Part model, mm, in its own coordinate system. A direction names the side the tool comes from. Coordinates: 2 decimals unless noted, no trailing zeros. Loops run counter-clockwise (first coordinate to the right, second up) from the corner with the lowest first, then second, coordinate; pieces in that order, holes last. Notation, with made-up numbers: (48.5, -22.5) - (90.5, -22.5) arc R13 cw to (90.5, -6.5) - close; hole circle Ø2 at (-22, 63). An arc over 180 degrees is marked (long way). Use a Markdown table: item, result. Add a question column.
1. Pull direction Z, two halves, no side cores. Call faces 4 (the flat face through (17, 30, 13)), 5 (the flat face through (73, 69, 3)), 6 (the cylindrical face through (57.846, 49.451, 7.93)): pulls with the +Z half, pulls with the -Z half, needs draft (parallel to the pull), parting line crosses it, or undercut.
2. Band-saw the part on D-D, the plane z = 19.5. Give the cut face in (x, y).
3. Band-saw the part on A-A, the plane x = 96. Give the cut face in (y, z).
4. Band-saw the part on C-C, the plane x = 154. Give the cut face in (y, z).
5. Wall check: probe 1 along Y at (x, z) = (8, 1.25); probe 2 along X at (y, z) = (29, 10); probe 3 along X at (y, z) = (56, 1). Give the ranges that are in metal, low to high. Write a range as [from, to].
6. 3-axis set-ups, long thin cutter, end or side, ignore diameter. For faces 1 (the flat face through (25, 98, 25)), 2 (the flat face through (56, 52, 13)), 3 (the cylindrical face through (107.05, 22.7, 7.93)): which of +Z, -Z, +X, -X, +Y, -Y reach the whole face in a straight line?
7. Band-saw the part on B-B, the plane x = 64.5. Give the cut face in (y, z).
8. Drop flat-ended pins along their axis: pin 1 (2 mm diameter, centred on x = 143, z = 41.5, fed in from +Y); pin 2 (1.5 mm diameter, centred on y = 67, z = 1.5, fed in from +X); pin 3 (21.5 mm diameter, centred on y = 92.5, z = 35.5, fed in from -X). Give the stop position or say it passes through.
from build123d import *

# Parameters (mm, degrees)
BOX006_W                  = 35
BOX006_H                  = 25
BOX006_DEPTH              = 10
CYLINDER010_R             = 0.7
CYLINDER010_DEPTH         = 10
CYLINDER011_R             = 4
CYLINDER011_DEPTH         = 10
CYLINDER012_R             = 0.7
CYLINDER012_DEPTH         = 10
CYLINDER013_R             = 4
CYLINDER013_DEPTH         = 10
CYLINDER009_R             = 0.7
CYLINDER009_DEPTH         = 10
CYLINDER008_R             = 4
CYLINDER008_DEPTH         = 10
CYLINDER016_R             = 0.7
CYLINDER016_DEPTH         = 10
CYLINDER017_R             = 4
CYLINDER017_DEPTH         = 10
CYLINDER018_R             = 0.7
CYLINDER018_DEPTH         = 10
CYLINDER019_R             = 4
CYLINDER019_DEPTH         = 10
FUSION003_PLACEMENT_ANGLE = 90
CYLINDER006_R             = 1
CYLINDER006_DEPTH         = 10
CYLINDER007_R             = 1
CYLINDER007_DEPTH         = 10
BOX005_W                  = 142
BOX005_H                  = 54
BOX005_DEPTH              = 3
CUT010_PLACEMENT_ANGLE    = 62
CYLINDER_R                = 1.5
CYLINDER_DEPTH            = 10
CYLINDER001_R             = 1.5
CYLINDER001_DEPTH         = 10
CYLINDER002_R             = 1.5
CYLINDER002_DEPTH         = 10
CYLINDER003_R             = 1.5
CYLINDER003_DEPTH         = 10
CYLINDER004_R             = 1.5
CYLINDER004_DEPTH         = 10
CYLINDER005_R             = 1.5
CYLINDER005_DEPTH         = 10
BOX004_W                  = 76
BOX004_H                  = 76
BOX004_DEPTH              = 10
BOX002_W                  = 192
BOX002_H                  = 72
BOX002_DEPTH              = 3
BOX003_W                  = 172
BOX003_H                  = 112
BOX003_DEPTH              = 3
BOX001_W                  = 192
BOX001_H                  = 112
BOX001_DEPTH              = 3
BOX_W                     = 192
BOX_H                     = 112
BOX_DEPTH                 = 3


with BuildPart() as cube006:
    # Box006 → Box006 (new body)
    with BuildSketch(Plane(origin=(81, 36, 0), x_dir=(1, 0, 0), z_dir=(0, 0, 1))):
        with Locations((17.5, 12.5)):
            Rectangle(BOX006_W, BOX006_H)
    extrude(amount=BOX006_DEPTH)


with BuildPart() as cylinder010:
    # Cylinder010 → Cylinder010 (new body)
    with BuildSketch(Plane.XY.offset(3)):
        Circle(CYLINDER010_R)
    extrude(amount=CYLINDER010_DEPTH)


with BuildPart() as cut012:
    # Cylinder011 → Cylinder011 (new body)
    with BuildSketch(Plane.XY.offset(3)):
        Circle(CYLINDER011_R)
    extrude(amount=CYLINDER011_DEPTH)

    # Cut012: cut Cylinder010
    add(cylinder010.part, mode=Mode.SUBTRACT)


with BuildPart() as cut012_1:
    # Cut012 placement: moved
    add(cut012.part.moved(Location((0, 34, 0))))


with BuildPart() as cylinder012:
    # Cylinder012 → Cylinder012 (new body)
    with BuildSketch(Plane.XY.offset(3)):
        Circle(CYLINDER012_R)
    extrude(amount=CYLINDER012_DEPTH)


with BuildPart() as cut013:
    # Cylinder013 → Cylinder013 (new body)
    with BuildSketch(Plane.XY.offset(3)):
        Circle(CYLINDER013_R)
    extrude(amount=CYLINDER013_DEPTH)

    # Cut013: cut Cylinder012
    add(cylinder012.part, mode=Mode.SUBTRACT)


with BuildPart() as cut013_1:
    # Cut013 placement: moved
    add(cut013.part.moved(Location((54, 1, 0))))


with BuildPart() as cylinder009:
    # Cylinder009 → Cylinder009 (new body)
    with BuildSketch(Plane.XY.offset(3)):
        Circle(CYLINDER009_R)
    extrude(amount=CYLINDER009_DEPTH)


with BuildPart() as fusion002:
    # Cylinder008 → Cylinder008 (new body)
    with BuildSketch(Plane.XY.offset(3)):
        Circle(CYLINDER008_R)
    extrude(amount=CYLINDER008_DEPTH)

    # Cut011: cut Cylinder009
    add(cylinder009.part, mode=Mode.SUBTRACT)

    # Fusion002: union Cut012, Cut013
    add(cut012_1.part)
    add(cut013_1.part)


with BuildPart() as fusion002_1:
    # Fusion002 placement: moved
    add(fusion002.part.moved(Location((56, 19, 0))))


with BuildPart() as cylinder016:
    # Cylinder016 → Cylinder016 (new body)
    with BuildSketch(Plane.XY.offset(3)):
        Circle(CYLINDER016_R)
    extrude(amount=CYLINDER016_DEPTH)


with BuildPart() as cut015:
    # Cylinder017 → Cylinder017 (new body)
    with BuildSketch(Plane.XY.offset(3)):
        Circle(CYLINDER017_R)
    extrude(amount=CYLINDER017_DEPTH)

    # Cut015: cut Cylinder016
    add(cylinder016.part, mode=Mode.SUBTRACT)


with BuildPart() as cut015_1:
    # Cut015 placement: moved
    add(cut015.part.moved(Location((0, 16, 0))))


with BuildPart() as cylinder018:
    # Cylinder018 → Cylinder018 (new body)
    with BuildSketch(Plane.XY.offset(3)):
        Circle(CYLINDER018_R)
    extrude(amount=CYLINDER018_DEPTH)


with BuildPart() as fusion003:
    # Cylinder019 → Cylinder019 (new body)
    with BuildSketch(Plane.XY.offset(3)):
        Circle(CYLINDER019_R)
    extrude(amount=CYLINDER019_DEPTH)

    # Cut016: cut Cylinder018
    add(cylinder018.part, mode=Mode.SUBTRACT)


with BuildPart() as fusion003_1:
    # Cut016 placement: moved
    add(fusion003.part.moved(Location((30, 0, 0))))

    # Fusion003: union Cut015
    add(cut015_1.part)


with BuildPart() as fusion003_2:
    # Fusion003 placement: moved
    add(fusion003_1.part.moved(Location((33, 29, 0))).rotate(Axis((33, 29, 0), (0, 0, 1)), FUSION003_PLACEMENT_ANGLE))


with BuildPart() as cylinder006:
    # Cylinder006 → Cylinder006 (new body)
    with BuildSketch(Plane(origin=(5, 8, 0), x_dir=(1, 0, 0), z_dir=(0, 0, 1))):
        Circle(CYLINDER006_R)
    extrude(amount=CYLINDER006_DEPTH)


with BuildPart() as cylinder007:
    # Cylinder007 → Cylinder007 (new body)
    with BuildSketch(Plane(origin=(137, 8, 0), x_dir=(1, 0, 0), z_dir=(0, 0, 1))):
        Circle(CYLINDER007_R)
    extrude(amount=CYLINDER007_DEPTH)


with BuildPart() as cut010:
    # Box005 → Box005 (new body)
    with BuildSketch(Plane.XY):
        with Locations((71, 27)):
            Rectangle(BOX005_W, BOX005_H)
    extrude(amount=BOX005_DEPTH)

    # Cut009: cut Cylinder007
    add(cylinder007.part, mode=Mode.SUBTRACT)

    # Cut010: cut Cylinder006
    add(cylinder006.part, mode=Mode.SUBTRACT)


with BuildPart() as cut010_1:
    # Cut010 placement: moved
    add(cut010.part.moved(Location((25, 86, 0))).rotate(Axis((25, 86, 0), (1, 0, 0)), CUT010_PLACEMENT_ANGLE))


with BuildPart() as cylinder:
    # Cylinder → Cylinder (new body)
    with BuildSketch(Plane(origin=(8, 56, 0), x_dir=(1, 0, 0), z_dir=(0, 0, 1))):
        Circle(CYLINDER_R)
    extrude(amount=CYLINDER_DEPTH)


with BuildPart() as cylinder001:
    # Cylinder001 → Cylinder001 (new body)
    with BuildSketch(Plane(origin=(8, 76, 0), x_dir=(1, 0, 0), z_dir=(0, 0, 1))):
        Circle(CYLINDER001_R)
    extrude(amount=CYLINDER001_DEPTH)


with BuildPart() as cylinder002:
    # Cylinder002 → Cylinder002 (new body)
    with BuildSketch(Plane(origin=(8, 36, 0), x_dir=(1, 0, 0), z_dir=(0, 0, 1))):
        Circle(CYLINDER002_R)
    extrude(amount=CYLINDER002_DEPTH)


with BuildPart() as cylinder003:
    # Cylinder003 → Cylinder003 (new body)
    with BuildSketch(Plane(origin=(15.75, 11, 0), x_dir=(1, 0, 0), z_dir=(0, 0, 1))):
        Circle(CYLINDER003_R)
    extrude(amount=CYLINDER003_DEPTH)


with BuildPart() as cylinder004:
    # Cylinder004 → Cylinder004 (new body)
    with BuildSketch(Plane(origin=(15.75, 101, 0), x_dir=(1, 0, 0), z_dir=(0, 0, 1))):
        Circle(CYLINDER004_R)
    extrude(amount=CYLINDER004_DEPTH)


with BuildPart() as cylinder005:
    # Cylinder005 → Cylinder005 (new body)
    with BuildSketch(Plane(origin=(176.25, 101, 0), x_dir=(1, 0, 0), z_dir=(0, 0, 1))):
        Circle(CYLINDER005_R)
    extrude(amount=CYLINDER005_DEPTH)


with BuildPart() as cube004:
    # Box004 → Box004 (new body)
    with BuildSketch(Plane(origin=(116, 0, 0), x_dir=(1, 0, 0), z_dir=(0, 0, 1))):
        with Locations((38, 38)):
            Rectangle(BOX004_W, BOX004_H)
    extrude(amount=BOX004_DEPTH)


with BuildPart() as cube002:
    # Box002 → Box002 (new body)
    with BuildSketch(Plane(origin=(0, 20, 0), x_dir=(1, 0, 0), z_dir=(0, 0, 1))):
        with Locations((96, 36)):
            Rectangle(BOX002_W, BOX002_H)
    extrude(amount=BOX002_DEPTH)


with BuildPart() as fusion:
    # Box003 → Box003 (new body)
    with BuildSketch(Plane(origin=(10, 0, 0), x_dir=(1, 0, 0), z_dir=(0, 0, 1))):
        with Locations((86, 56)):
            Rectangle(BOX003_W, BOX003_H)
    extrude(amount=BOX003_DEPTH)

    # Fusion: union Cube002
    add(cube002.part)


with BuildPart() as cut:
    # Box001 → Box001 (new body)
    with BuildSketch(Plane.XY):
        with Locations((96, 56)):
            Rectangle(BOX001_W, BOX001_H)
    extrude(amount=BOX001_DEPTH)

    # Cut: cut Fusion
    add(fusion.part, mode=Mode.SUBTRACT)


with BuildPart() as cut017:
    # Box → Box (new body)
    with BuildSketch(Plane.XY):
        with Locations((96, 56)):
            Rectangle(BOX_W, BOX_H)
    extrude(amount=BOX_DEPTH)

    # Cut001: cut Cut
    add(cut.part, mode=Mode.SUBTRACT)

    # Cut002: cut Cube004
    add(cube004.part, mode=Mode.SUBTRACT)

    # Cut003: cut Cylinder005
    add(cylinder005.part, mode=Mode.SUBTRACT)

    # Cut004: cut Cylinder004
    add(cylinder004.part, mode=Mode.SUBTRACT)

    # Cut005: cut Cylinder003
    add(cylinder003.part, mode=Mode.SUBTRACT)

    # Cut006: cut Cylinder002
    add(cylinder002.part, mode=Mode.SUBTRACT)

    # Cut007: cut Cylinder001
    add(cylinder001.part, mode=Mode.SUBTRACT)

    # Cut008: cut Cylinder
    add(cylinder.part, mode=Mode.SUBTRACT)

    # Fusion001: union Cut010
    add(cut010_1.part)

    # Fusion004: union Fusion002, Fusion003
    add(fusion002_1.part)
    add(fusion003_2.part)

    # Cut017: cut Cube006
    add(cube006.part, mode=Mode.SUBTRACT)


solid = cut017.part
Geometry check:
| question | item | result |
|---|---|---|
| 1 | face 4 | pulls with the +Z half |
| 1 | face 5 | undercut |
| 1 | face 6 | needs draft |
| 2 | outline | (25, 92.97) - (167, 92.97) - (167, 96.37) - (25, 96.37) - close |
| 3 | outline | (0, 0) - (36, 0) - (36, 3) - (0, 3) - close; (61, 0) - (112, 0) - (112, 3) - (87.6, 3) - (111.35, 47.68) - (108.7, 49.09) - (84.2, 3) - (61, 3) - close |
| 4 | outline | (76, 0) - (112, 0) - (112, 3) - (87.6, 3) - (111.35, 47.68) - (108.7, 49.09) - (84.2, 3) - (76, 3) - close |
| 5 | probe 1 | y = [20, 34.5], [37.5, 54.5], [57.5, 74.5], [77.5, 92] |
| 5 | probe 2 | x = [13, 16.3], [17.7, 21] |
| 5 | probe 3 | x = [0, 6.5], [9.5, 81] |
| 6 | face 1 | +Z, -X, +Y, -Y |
| 6 | face 2 | +Z, +X, -X, -Y |
| 6 | face 3 | +Z |
| 7 | outline | (0, 0) - (112, 0) - (112, 3) - (87.6, 3) - (111.35, 47.68) - (108.7, 49.09) - (84.2, 3) - (0, 3) - close |
| 8 | pin 1 | stops at y = 108.6 |
| 8 | pin 2 | stops at x = 116 |
| 8 | pin 3 | stops at x = 25 |
